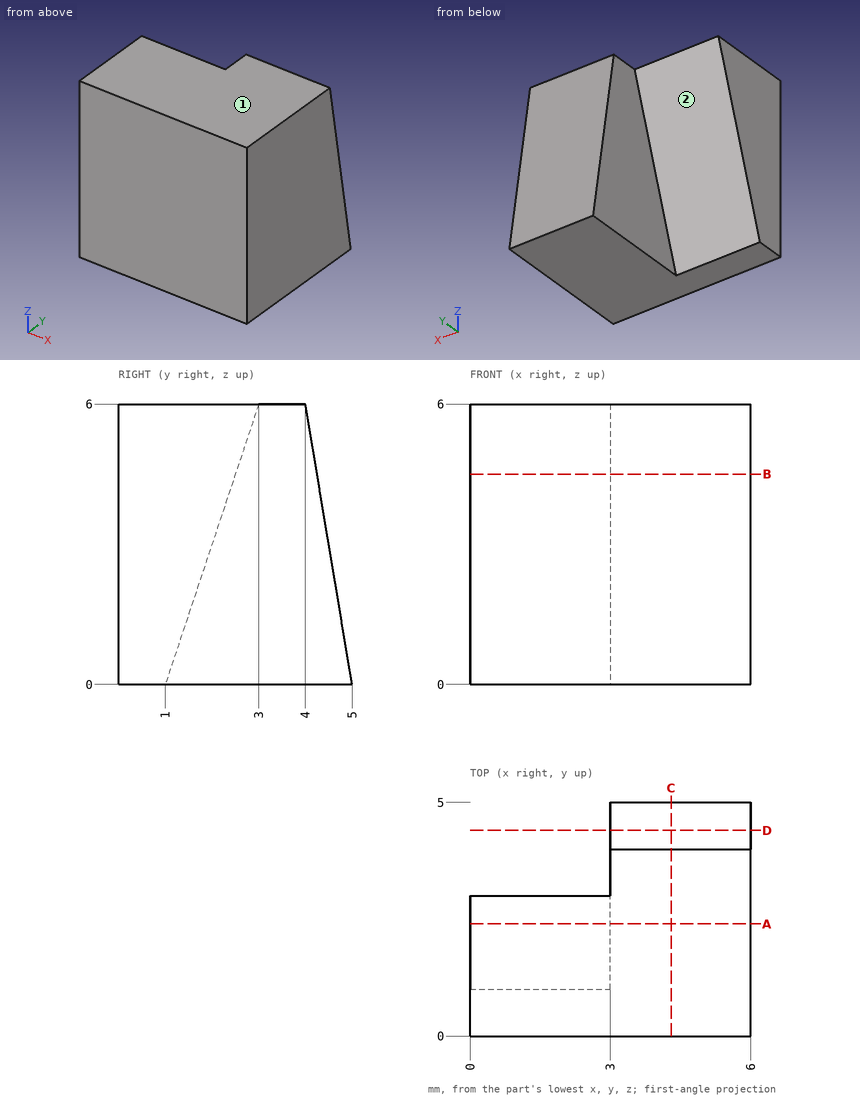
Part print with two shaded views. Sizes in mm from the minimum x, y, z corner. A direction names the side the tool comes from. Coordinates: 2 decimals unless noted, no trailing zeros. Write each loop counter-clockwise with the first axis right and the second up, starting at its lowest first coordinate (ties: lowest second). Pieces come first, ordered by that corner, then holes.
(1) Cut at B-B on z = 4.5. List the corners of the cut face in (x, y).
(2) 3-axis set-ups, long thin cutter, end or side, ignore diameter. For the marked faces 1 and 2: which of +Z, -Z, +X, -X, +Y, -Y reach the whole face in a straight line?
(3) Cut at A-A on y = 2.4. List the corners of the cut face in (x, z), and give its area (3 significant figures).
(4) Pin check, flat tips, straight feed: pin 1 Ø1 at (x, z) = (5, 4.5) entering from +Y; pin 2 Ø1.2 at (y, z) = (3, 3.5) entering from -X; pin 3 Ø1.5 at (x, z) = (3.5, 2) entering from +Y. Stop position of each tip, or through.
(5) Drill centre lines: line 1 (X direction, y = 2.3, z = 0.75); line 2 (Y direction, x = 2, z = 2.5); line 3 (Y direction, x = 5.7, z = 4.75). Where is each one in solid material? Low to high.
(6) Cut at C-C on x = 4.3. List the corners of the cut face in (y, z).
(7) Cut at D-D on y = 4.4. List the corners of the cut face in (x, z), and give its area (3 significant figures).
Working result:
1. outline: (0, 0) - (6, 0) - (6, 4.25) - (3, 4.25) - (3, 2.5) - (0, 2.5) - close
2. face 1: +Z, +X, -X, +Y, -Y
2. face 2: -Z, -X, +Y
3. outline: (0, 4.2) - (3, 4.2) - (3, 0) - (6, 0) - (6, 6) - (0, 6) - close
3. area: 23.4 mm2
4. pin 1: stops at y = 4.33
4. pin 2: stops at x = 3
4. pin 3: stops at y = 4.79
5. line 1: x = 3 to 6
5. line 2: y = 0 to 1.83
5. line 3: y = 0 to 4.21
6. outline: (0, 0) - (5, 0) - (4, 6) - (0, 6) - close
7. outline: (3, 0) - (6, 0) - (6, 3.6) - (3, 3.6) - close
7. area: 10.8 mm2
